Input: part model. Units: mm. Frame: model coordinates. A direction names the side the tool comes from. Give positions to 0.01 mm unless a question says otherwise; leave off trailing zeros. Write each loop counter-clockwise with the first axis right and the second up, starting at its lowest first coordinate (ties: lowest second). Pieces come first, ordered by that corner, then holes. Notation, with made-up numbers: (9.5, 21) -> (40.5, 21) arc R25 ccw to (40.5, 57) -> close; hole circle Ø4 at (-20, 68). An arc over 180 degrees is marked (long way). Return JSON: item names as keys, results as strings. Group by question number.
Item 1: Section C-C, the plane x = 1444. Return loops of the section in (y, z).
Item 2: Set-up query: faces 1 (the face through (1417.39, -572.95, 54.58)), 2 (the face through (435, -578, 85)), 3 (the face through (1260.564, -457.042, 43.095)). Return all of +Z, -Z, +X, -X, +Y, -Y with unobstructed straight access to the full face (end or side cutting, diameter ignored); none if empty.
Item 3: Mould query, pull axis Y, two halves, no side actions, for faces 4 (the face through (1127, -664, 0)), 5 (the face through (1704, 0, 34)), 6 (the face through (444.892, -589.216, 54.58)). Classes: released by +Y, released by -Y, zero draft, split by the parting line, or undercut.
Item 4: Section A-A, the plane z = 50. Return loops of the section in (x, y).
Item 5: Line query: line 1 (X direction, y = -318, z = 52); line 2 (X direction, y = -54, z = 48); line 3 (Z direction, x = 1359, y = -577). Output: solid intervals per line, ascending. Write a range as [from, to].
Item 6: Pin query (flat end, axial travel): P1, Ø5, axis at x = 1438, z = 76.5, coming from the -Y side; P2, Ø10, axis at x = 956.5, z = 40.5, coming from the -Y side; P3, Ø1.5, axis at x = 1346, z = 48.5, coming from the +Y side. Return the tip coordinate at first contact, or that it passes through.
Item 7: Section B-B, the plane y = -856. Return loops of the section in (x, z), then the cut area to 3 significant figures.
Item 8: Section D-D, the plane x = 222.5. Return loops of the section in (y, z).
from build123d import *

# Parameters (mm, degrees)
F1_DEPTH      = 25
F3_DEPTH      = 60
F5_DEPTH      = 60
F5_DEPTH_BACK = 25
F7_DEPTH      = 85.001


with BuildPart() as f1:
    # F0 (on Top) → F1 (new body)
    with BuildSketch(Plane.XY):
        Polygon((1850, 0), (0, 0), (877.5, -1162.1623567633), (972.5, -1162.1623567633), align=None)
    extrude(amount=F1_DEPTH)

    # F2 (on face) → F3 (join)
    with BuildSketch(Plane.XY.offset(25)):
        Polygon((119.0389274289, 0), (925, -1067.4160906651), (1730.9610725711, 0), align=None)
    extrude(amount=F3_DEPTH)

    # F4 (on face) → F5 (join, two sides)
    with BuildSketch(Plane.XY.offset(25)) as f5_sk:
        Polygon((-3.7591240241, 0), (873.7408759759, -1162.1623567633), (877.5, -1162.1623567633), (0, 0), align=None)
        Polygon((1850, 0), (972.5, -1162.1623567633), (976.2591240241, -1162.1623567633), (1853.7591240241, 0), align=None)
    extrude(amount=F5_DEPTH)
    extrude(f5_sk.sketch, amount=-F5_DEPTH_BACK)

    # F6 (on face) → F7 (cut, through all)
    with BuildSketch(Plane.XY.offset(85)):
        Polygon((244.3430615646, 0), (925, -901.4631016744), (1605.6569384354, 0), align=None)
    extrude(amount=-F7_DEPTH, mode=Mode.SUBTRACT)


solid = f1.part
Answer below:
{
 "1": {"outline": "(-542.69, 0) -> (-214.1, 0) -> (-214.1, 85) -> (-380.05, 85) -> (-380.05, 25) -> (-537.71, 25) -> (-537.71, 85) -> (-542.69, 85) -> close"},
 "2": {"face 1": "+Z", "face 2": "+Z, +X, -X, +Y, -Y", "face 3": "+Z, -Z, +Y"},
 "3": {"face 4": "zero draft", "face 5": "released by +Y", "face 6": "undercut"},
 "4": {"outline": "(-3.76, 0) -> (873.74, -1162.16) -> (877.5, -1162.16) -> (0, 0) -> close; (119.04, 0) -> (925, -1067.42) -> (1730.96, 0) -> (1605.66, 0) -> (925, -901.46) -> (244.34, 0) -> close; (972.5, -1162.16) -> (976.26, -1162.16) -> (1853.76, 0) -> (1850, 0) -> close"},
 "5": {"line 1": "x = [236.35, 240.11], [359.15, 484.45], [1365.55, 1490.85], [1609.89, 1613.65]", "line 2": "x = [37.01, 40.77], [159.81, 285.12], [1564.88, 1690.19], [1809.23, 1812.99]", "line 3": "z = [0, 25]"},
 "6": {"P1": "stops at y = -553.94", "P2": "stops at y = -1032.32", "P3": "stops at y = -342.9"},
 "7": {"outline": "(642.57, 0) -> (890.67, 0) -> (890.67, 85) -> (765.37, 85) -> (765.37, 25) -> (646.33, 25) -> (646.33, 85) -> (642.57, 85) -> close; (959.33, 0) -> (1207.43, 0) -> (1207.43, 85) -> (1203.67, 85) -> (1203.67, 25) -> (1084.63, 25) -> (1084.63, 85) -> (959.33, 85) -> close", "area": "27,900 mm2"},
 "8": {"outline": "(-299.66, 0) -> (0, 0) -> (0, 85) -> (-137.02, 85) -> (-137.02, 25) -> (-294.68, 25) -> (-294.68, 85) -> (-299.66, 85) -> close"}
}
